Part model, mm, in its own coordinate system. A direction names the side the tool comes from. Round coordinates to 2 decimals unless told otherwise and drop trailing zeros. Loops run counter-clockwise (first coordinate to the right, second up) from the corner with the lowest first, then second, coordinate; pieces in that order, holes last. Notation, with made-up numbers: (62, -31.75) -> (119, -31.75) arc R29 ccw to (119, -11.75) -> close; hole circle Ø8 at (28, 81.5). An arc over 180 degrees is marked (long way). Answer as CSV lines item,"result".
from build123d import *

# Parameters (mm, degrees)
SKETCH1_W           = 32
SKETCH1_H           = 32
BOSS_EXTRUDE1_DEPTH = 0.681
SKETCH2_R           = 1.3335
CUT_EXTRUDE1_DEPTH  = 1
FILLET1_R           = 1.335
SKETCH3_R           = 1.4285
SKETCH3_W           = 20.57
SKETCH3_H           = 20.57
BOSS_EXTRUDE2_DEPTH = 2.857
SKETCH4_R           = 8.1405
BOSS_EXTRUDE3_DEPTH = 17.46
SKETCH6_R           = 5.6075
CUT_EXTRUDE2_DEPTH  = 2


with BuildPart() as part:
    # Sketch1 → Boss-Extrude1 (new body)
    with BuildSketch(Plane(origin=(0, 0, 0), x_dir=(1, 0, 0), z_dir=(0, 1, 0))):
        Rectangle(SKETCH1_W, SKETCH1_H)
    extrude(amount=BOSS_EXTRUDE1_DEPTH)

    # Sketch2 → Cut-Extrude1 (cut)
    with BuildSketch(Plane(origin=(0, 0.681, 0), x_dir=(1, 0, 0), z_dir=(0, 1, 0))):
        with Locations(Location((13.75, 13.75, 0), (0, 0, 270))):
            Circle(SKETCH2_R)
        with Locations(Location((-13.75, 13.75, 0), (0, 0, 270))):
            Circle(SKETCH2_R)
        with Locations(Location((-13.75, -13.75, 0), (0, 0, 270))):
            Circle(SKETCH2_R)
        with Locations(Location((13.75, -13.75, 0), (0, 0, 270))):
            Circle(SKETCH2_R)
    extrude(amount=-CUT_EXTRUDE1_DEPTH, mode=Mode.SUBTRACT)

    # Fillet1
    fillet1_edges = [part.edges().sort_by_distance(p)[0] for p in [
        (16, 0.3405, 16),
        (-16, 0.3405, 16),
        (-16, 0.3405, -16),
        (16, 0.3405, -16),
    ]]
    fillet(fillet1_edges, radius=FILLET1_R)

    # Sketch3 → Boss-Extrude2 (add)
    with BuildSketch(Plane(origin=(0, 0.681, 0), x_dir=(1, 0, 0), z_dir=(0, 1, 0))):
        with Locations((0, -10.857)):
            Circle(SKETCH3_R)
        with Locations((0, 10.857)):
            Circle(SKETCH3_R)
        Rectangle(SKETCH3_W, SKETCH3_H)
        with BuildLine():
            ThreePointArc((1.308979851, -10.285), (0, -9.4285), (-1.308979851, -10.285))
            Line((-1.308979851, -10.285), (1.308979851, -10.285))
        make_face()
        with BuildLine():
            Line((1.308979851, -10.285), (-1.308979851, -10.285))
            ThreePointArc((-1.308979851, -10.285), (-1.398300749, -10.564823227), (-1.4285, -10.857))
            ThreePointArc((-1.4285, -10.857), (0, -12.2855), (1.4285, -10.857))
            ThreePointArc((1.4285, -10.857), (1.398300749, -10.564823227), (1.308979851, -10.285))
        make_face()
        with BuildLine():
            Line((1.4285, -10.285), (1.308979851, -10.285))
            ThreePointArc((1.308979851, -10.285), (1.398300749, -10.564823227), (1.4285, -10.857))
            Line((1.4285, -10.857), (1.4285, -10.285))
        make_face()
        with BuildLine():
            Line((-1.308979851, -10.285), (-1.4285, -10.285))
            Line((-1.4285, -10.285), (-1.4285, -10.857))
            ThreePointArc((-1.4285, -10.857), (-1.398300749, -10.564823227), (-1.308979851, -10.285))
        make_face()
        with BuildLine():
            ThreePointArc((-1.4285, 10.857), (-1.398300749, 10.564823227), (-1.308979851, 10.285))
            Line((-1.308979851, 10.285), (1.308979851, 10.285))
            ThreePointArc((1.308979851, 10.285), (1.398300749, 10.564823227), (1.4285, 10.857))
            ThreePointArc((1.4285, 10.857), (0, 12.2855), (-1.4285, 10.857))
        make_face()
        with BuildLine():
            Line((1.308979851, 10.285), (-1.308979851, 10.285))
            ThreePointArc((-1.308979851, 10.285), (0, 9.4285), (1.308979851, 10.285))
        make_face()
        with BuildLine():
            ThreePointArc((1.4285, 10.857), (1.398300749, 10.564823227), (1.308979851, 10.285))
            Line((1.308979851, 10.285), (1.4285, 10.285))
            Line((1.4285, 10.285), (1.4285, 10.857))
        make_face()
        with BuildLine():
            Line((-1.4285, 10.857), (-1.4285, 10.285))
            Line((-1.4285, 10.285), (-1.308979851, 10.285))
            ThreePointArc((-1.308979851, 10.285), (-1.398300749, 10.564823227), (-1.4285, 10.857))
        make_face()
    extrude(amount=BOSS_EXTRUDE2_DEPTH)

    # Sketch4 → Boss-Extrude3 (add)
    with BuildSketch(Plane(origin=(0, 3.538, 0), x_dir=(1, 0, 0), z_dir=(0, 1, 0))):
        with Locations(Location((0, 0, 0), (0, 0, 270))):
            Circle(SKETCH4_R)
    extrude(amount=BOSS_EXTRUDE3_DEPTH)

    # Sketch6 → Cut-Extrude2 (cut)
    with BuildSketch(Plane(origin=(0, 20.998, 0), x_dir=(1, 0, 0), z_dir=(0, 1, 0))):
        with Locations(Location((0, 0, 0), (0, 0, 270))):
            Circle(SKETCH6_R)
    extrude(amount=-CUT_EXTRUDE2_DEPTH, mode=Mode.SUBTRACT)


solid = part.part
Q1. Saw through at D-D, the plane y = 9.75. Write the cut outline in (x, z), then the cut area to 3 significant figures.
Geometry results:
outline,"circle Ø16.28 at (0, 0)"
area,"208 mm2"
Q2. Drill centre lines: line 1 along X through (y, z) = (0.55, -13.75); line 2 along X through (y, z) = (19.6, 0); line 3 along Y through (x, z) = (10, 11). Where is each one in solid material? Low to high.
Geometry results:
line 1,"-16 to -15.08, -12.42 to 12.42, 15.08 to 16"
line 2,"-8.14 to -5.61, 5.61 to 8.14"
line 3,"0 to 0.68"
Q3. Two-plate mould, pull along Z, no slides. Class faces 4 (the face through (13.809, 0.345, -15.082)), 5 (the face through (10.285, 2, 0)), 6 (the face through (6.86, 12.15, 4.38)): pulls with the +Z half, pulls with the -Z half, needs draft (parallel to the pull), parting line crosses it, or undercut.
Geometry results:
face 4,"undercut"
face 5,"needs draft"
face 6,"parting line crosses it"
Q4. Which spindle directions (+Z, -Z, +X, -X, +Y, -Y) get a long thin tool onto all of the face, cutting with end or side? Do faces 1 (the face through (6, 2, 10.285)), 2 (the face through (0.031, 2.09, -12.285)), 3 (the face through (-6, 2, -10.285)). Say none if no direction does.
Geometry results:
face 1,"+Z, +X, +Y"
face 2,"-Z, +Y"
face 3,"-Z, -X, +Y"
Q5. Saw through at B-B, the plane z = -13.75. Write the cut outline in (x, y), then the cut area to 3 significant figures.
Geometry results:
outline,"(-16, 0) -> (-15.08, 0) -> (-15.08, 0.68) -> (-16, 0.68) -> close; (-12.42, 0) -> (12.42, 0) -> (12.42, 0.68) -> (-12.42, 0.68) -> close; (15.08, 0) -> (16, 0) -> (16, 0.68) -> (15.08, 0.68) -> close"
area,"18.2 mm2"
Q6. Drop flat-ended pins along their axis: P1, Ø8, axis at x = -7.5, y = 15, coming from the +Z side; P2, Ø1.4, axis at x = 8, y = 2, coming from the +Z side (3 decimals); P3, Ø1.5, axis at x = -8, z = -12, coming from the -Y side; P4, Ø6, axis at x = -1.5, y = 5, coming from the +Z side. Give the stop position or say it passes through.
Geometry results:
P1,"z = 7.35"
P2,"z = 10.285"
P3,"y = 0"
P4,"z = 12.29"
Q7. Saw through at A-A, the plane x = 13.75. Write the cut outline in (y, z).
Geometry results:
outline,"(0, -16) -> (0.68, -16) -> (0.68, -15.08) -> (0, -15.08) -> close; (0, -12.42) -> (0.68, -12.42) -> (0.68, 12.42) -> (0, 12.42) -> close; (0, 15.08) -> (0.68, 15.08) -> (0.68, 16) -> (0, 16) -> close"
Q8. Saw through at C-C, the plane x = 0. Write the cut outline in (y, z).
Geometry results:
outline,"(0, -16) -> (0.68, -16) -> (0.68, -12.29) -> (3.54, -12.29) -> (3.54, -8.14) -> (21, -8.14) -> (21, -5.61) -> (19, -5.61) -> (19, 5.61) -> (21, 5.61) -> (21, 8.14) -> (3.54, 8.14) -> (3.54, 12.29) -> (0.68, 12.29) -> (0.68, 16) -> (0, 16) -> close"
